Check sheet for the modelled part. Datum: model origin and axes. Units: mm. Face numbers are marked on the shaded views. Coordinates: 2 decimals unless noted, no trailing zeros. Answer as CSV lines item,"result".
from build123d import *

# Parameters (mm, degrees)
SKETCH1_W             = 633.5522
SKETCH1_H             = 50.8
BOSS_EXTRUDE1_DEPTH   = 0.79375
FILLET1_R             = 6.35
F_6_CLEARANCE_HOLE1_D = 3.7973


with BuildPart() as part:
    # Sketch1 → Boss-Extrude1 (new body)
    with BuildSketch(Plane(origin=(0, 0, 0), x_dir=(1, 0, 0), z_dir=(0, 1, 0))):
        Rectangle(SKETCH1_W, SKETCH1_H)
    extrude(amount=BOSS_EXTRUDE1_DEPTH)

    # Fillet1
    fillet1_edges = [part.edges().sort_by_distance(p)[0] for p in [
        (316.7761, 0.396875, 25.4),
        (-316.7761, 0.396875, 25.4),
        (-316.7761, 0.396875, -25.4),
        (316.7761, 0.396875, -25.4),
    ]]
    fillet(fillet1_edges, radius=FILLET1_R)

    # #6 Clearance Hole1 (through all)
    with Locations(Plane(origin=(0, 0.79375, 0), x_dir=(1, 0, 0), z_dir=(0, 1, 0))):
        with Locations((294.256791216, 0), (0, 0), (-294.256791216, 0)):
            Hole(F_6_CLEARANCE_HOLE1_D / 2)


solid = part.part
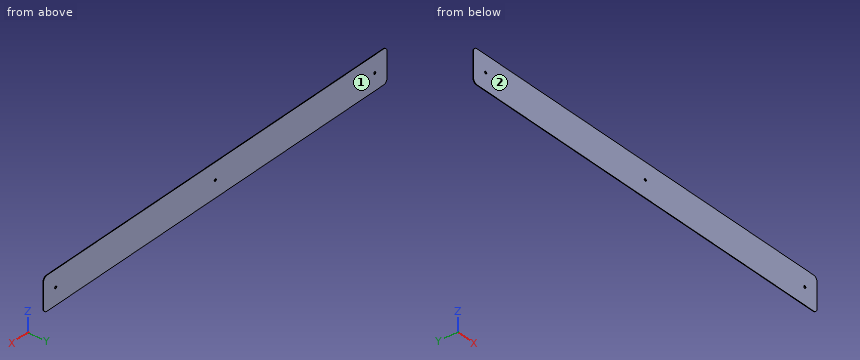
1) Mould release check, pull along Y, two halves, no side actions. Record for the marked faces 1 and 2: pulls with the +Y half, pulls with the -Y half, needs draft (parallel to the pull), parting line crosses it, or undercut.
Answer key:
face 1,"pulls with the +Y half"
face 2,"pulls with the -Y half"
2) Thickness scan on line 1 along X through (y, z) = (0.2, 1.5); line 2 along Z through (x, y) = (0, 0.35); line 3 along X through (y, z) = (0.7, 23). Record the ranges inside material, lowest first.
Answer key:
line 1,"x = -316.78 to -295.42, -293.09 to -1.16, 1.16 to 293.09, 295.42 to 316.78"
line 2,"z = -25.4 to -1.9, 1.9 to 25.4"
line 3,"x = -315.4 to 315.4"
3) Depth check by flat-ended pin: P1, Ø2, axis at x = -171.5, z = 13.5, coming from the -Y side. Enter the tip coordinate at first touch or a pass-through.
Answer key:
P1,"stops at y = 0"
